```python
from build123d import *

# Parameters (mm, degrees)
F0_W     = 68.5
F0_H     = 30.3
F1_DEPTH = 30.8
F2_R     = 7.9
F3_DEPTH = 3.7
F4_R     = 7
F5_DEPTH = 6.5
F7_D     = 5.5
F8_R     = 3
F9_DEPTH = 8
F10_R    = 1


with BuildPart() as f1:
    # F0 (on Top) → F1 (new body)
    with BuildSketch(Plane.XY):
        Rectangle(F0_W, F0_H)
    extrude(amount=F1_DEPTH)

    # F2 (on face) → F3 (join)
    with BuildSketch(Plane(origin=(-34.25, 0, 0), x_dir=(0, -1, 0), z_dir=(-1, 0, 0))):
        with Locations((0, 14.9)):
            Circle(F2_R)
    extrude(amount=F3_DEPTH)

    # F4 (on face) → F5 (join)
    with BuildSketch(Plane.YZ.offset(34.25)):
        with Locations((0, 15.4)):
            Circle(F4_R)
    extrude(amount=F5_DEPTH)

    # F7 (through all)
    with Locations(Plane(origin=(0, 15.15, 0), x_dir=(-1, 0, 0), z_dir=(0, 1, 0))):
        with Locations((28.8861435714, 26.8), (28.8861435714, 4)):
            Hole(F7_D / 2)

    # F8 (on face) → F9 (join)
    with BuildSketch(Plane(origin=(-37.95, 0, 0), x_dir=(0, -1, 0), z_dir=(-1, 0, 0))):
        with Locations((0, 14.9)):
            Circle(F8_R)
    extrude(amount=F9_DEPTH)

    # F10
    f10_edges = [f1.edges().sort_by_distance(p)[0] for p in [
        (-45.95, 3, 14.9),
    ]]
    fillet(f10_edges, radius=F10_R)


solid = f1.part
```
Input: part model. Units: mm. Frame: model coordinates. A direction names the side the tool comes from. Coordinates: 2 decimals unless noted, no trailing zeros. Write each loop counter-clockwise with the first axis right and the second up, starting at its lowest first coordinate (ties: lowest second). Pieces come first, ordered by that corner, then holes.
1) Mould query, pull axis Z, two halves, no side actions, for faces 1 (the flat face through (-37.95, -3.4, 15)), 2 (the cylindrical face through (-36.074, 1.713, 7.188)), 3 (the cylindrical face through (-29.482, -0.212, 1.315)), 4 (the cylindrical face through (-29.482, -0.212, 24.115)). Classes: pulls with the +Z half, pulls with the -Z half, needs draft (parallel to the pull), parting line crosses it, or undercut.
2) Section B-B on z = 4. Output: boundary loops of the cut face in (x, y), and give its area (3 significant figures).
3) Material intervals for line 1 along X through (y, z) = (2, 8); line 2 along X through (y, z) = (2, 22); line 3 along X through (y, z) = (8, 29), sorted ascending.
4) Section D-D on x = -39.5. Output: boundary loops of the cut face in (y, z).
5) Section C-C on y = 5. Output: boundary loops of the cut face in (x, z), and give its area (3 significant figures).
6) Section A-A on y = 0. Output: boundary loops of the cut face in (x, z).
7) Set-up query: faces 5 (the flat face through (0, 0, 30.8)), 6 (the cylindrical face through (37.45, -0.91, 22.34)), 7 (the flat face through (-34.25, -4, 22)). Return all of +Z, -Z, +X, -X, +Y, -Y with unobstructed straight access to the full face (end or side cutting, diameter ignored); none if empty.
8) Pin query (flat end, axial travel): pin 1 Ø2 at (y, z) = (2.5, 9.5) entering from -X; pin 2 Ø6 at (x, y) = (32, -5.5) entering from -Z; pin 3 Ø3.5 at (x, z) = (-28.89, 26.8) entering from -Y. Return the tip coordinate at first contact, or that it passes through.
Check result:
1. face 1: needs draft
1. face 2: parting line crosses it
1. face 3: undercut
1. face 4: undercut
2. outline: (-34.25, -15.15) - (-31.64, -15.15) - (-31.64, 15.15) - (-34.25, 15.15) - close; (-26.14, -15.15) - (34.25, -15.15) - (34.25, 15.15) - (-26.14, 15.15) - close
2. area: 1,910 mm2
3. line 1: x = -37.95 to 34.25
3. line 2: x = -37.95 to 40.75
3. line 3: x = -34.25 to -30.54, -27.24 to 34.25
4. outline: circle Ø6 at (0, 14.9)
5. outline: (-37.95, 8.78) - (-34.25, 8.78) - (-34.25, 0) - (34.25, 0) - (34.25, 10.5) - (40.75, 10.5) - (40.75, 20.3) - (34.25, 20.3) - (34.25, 30.8) - (-34.25, 30.8) - (-34.25, 21.02) - (-37.95, 21.02) - close; hole circle Ø5.5 at (-28.89, 4); hole circle Ø5.5 at (-28.89, 26.8)
5. area: 2,170 mm2
6. outline: (-45.95, 12.9) arc R1 ccw to (-44.95, 11.9) - (-37.95, 11.9) - (-37.95, 7) - (-34.25, 7) - (-34.25, 0) - (34.25, 0) - (34.25, 8.4) - (40.75, 8.4) - (40.75, 22.4) - (34.25, 22.4) - (34.25, 30.8) - (-34.25, 30.8) - (-34.25, 22.8) - (-37.95, 22.8) - (-37.95, 17.9) - (-44.95, 17.9) arc R1 ccw to (-45.95, 16.9) - close; hole circle Ø5.5 at (-28.89, 4); hole circle Ø5.5 at (-28.89, 26.8)
7. face 5: +Z, +X, -X, +Y, -Y
7. face 6: +X
7. face 7: -X
8. pin 1: stops at x = -37.95
8. pin 2: stops at z = 0
8. pin 3: passes through
